Check sheet for the drawn part. Datum: minimum x, y, z corner. Units: mm. Coordinates: 2 decimals unless noted, no trailing zeros. Loops run counter-clockwise (first coordinate to the right, second up) from the corner with the lowest first, then second, coordinate; pieces in that order, holes last. Notation, with made-up numbers: (66.5, 88.25) - (73.5, 88.25) arc R25 cw to (73.5, 118.25) - close; hole circle Ø5 at (53, -39.75). An arc over 180 degrees is marked (long way). Write item = value, one per line. Start each with the question number.
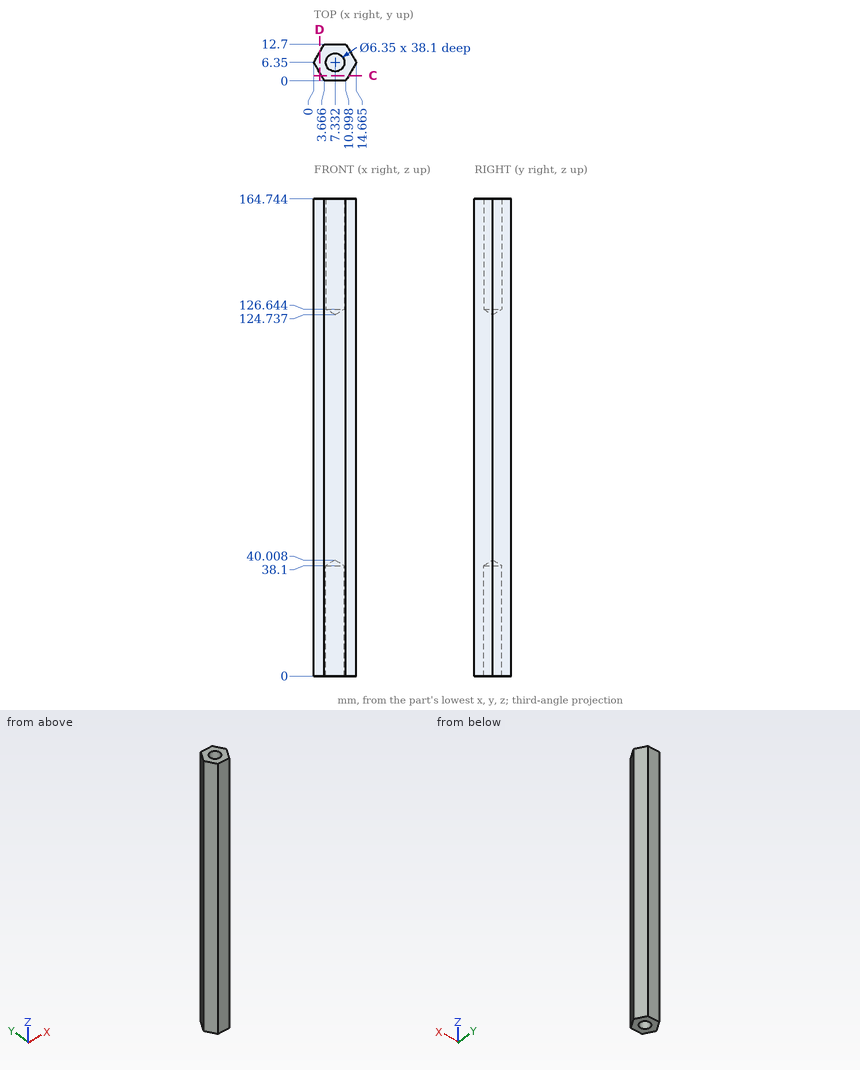
(1) Scan lines: line 1 (Y direction, x = 11, z = 147.5) (1 decimal); line 2 (Y direction, x = 9, z = 153); line 3 (Y direction, x = 14.25, z = 101) (1 decimal). Record each from-to range of solid material in increasing order.
(2) Sectioned sample at D-D on x = 2. Enter the section's corners in (y, z) (1 decimal).
(3) Depth check by flat-ended pin: pin 1 (1.5 mm diameter, centred on y = 2.5, z = 109.5, fed in from -X); pin 2 (5 mm diameter, centred on x = 2.5, z = 42.5, fed in from -Y); pin 3 (4 mm diameter, centred on x = 7.33, y = 6.35, fed in from -Z) (1 decimal); pin 4 (5.5 mm diameter, centred on x = 7.33, y = 6.35, fed in from +Z). Enter the tip coordinate at first touch or a pass-through.
(4) Sectioned sample at C-C on y = 1.75. Enter the section's corners in (x, z) (1 decimal).
Working result:
q1.line_1 = 0 to 12.7
q1.line_2 = 0 to 3.65, 9.05 to 12.7
q1.line_3 = 5.6 to 7.1
q2.outline = (2.9, 0) - (9.8, 0) - (9.8, 164.7) - (2.9, 164.7) - close
q3.pin_1 = 1.79
q3.pin_2 = 0
q3.pin_3 = 38.8
q3.pin_4 = 126.39
q4.outline = (2.7, 0) - (12, 0) - (12, 164.7) - (2.7, 164.7) - close
